```python
from build123d import *

# Parameters (mm, degrees)
F1_DEPTH = 1.85
F2_W     = 0.5
F2_H     = 21
F3_DEPTH = 3
F4_R     = 1.75
F5_DEPTH = 1.851
F6_W     = 0.25
F6_H     = 3.7
F7_DEPTH = 0.25
F8_R     = 0.24999
F9_R     = 0.4999
F10_R    = 0.24999


# Not quite as in the source:
# - a fillet or chamfer is up to 0.001 mm smaller than in the source, because OpenCascade refuses the exact size


with BuildPart() as f1:
    # F0 (on Right) → F1 (new body)
    with BuildSketch(Plane.YZ):
        Polygon((0, 9.2), (0, 0), (23.5, 0), (23.5, 13.7), (2.5, 13.7), (2.5, 9.2), align=None)
    extrude(amount=F1_DEPTH)

    # F2 (on face) → F3 (join)
    with BuildSketch(Plane.XY.offset(13.7)):
        with Locations((0.25, 13)):
            Rectangle(F2_W, F2_H)
    extrude(amount=F3_DEPTH)

    # F4 (on face) → F5 (cut, through all)
    with BuildSketch(Plane.YZ.offset(1.85)):
        with Locations((6, 3.1)):
            Circle(F4_R)
        with Locations((15, 3.1)):
            Circle(F4_R)
    extrude(amount=-F5_DEPTH, mode=Mode.SUBTRACT)

    # F6 (on face) → F7 (join)
    with BuildSketch(Plane(origin=(0, 0, 0), x_dir=(0, -1, 0), z_dir=(-1, 0, 0))):
        with Locations((-15.375, 14.85)):
            Rectangle(F6_W, F6_H)
        with Locations((-10.625, 14.85)):
            Rectangle(F6_W, F6_H)
    extrude(amount=F7_DEPTH)

    # F8 (radius 0.25 in the source; OpenCascade refuses exactly that, so slightly less here)
    f8_edges = [f1.edges().sort_by_distance(p)[0] for p in [
        (0, 6.5, 16.7),
        (0, 13, 16.7),
        (0, 19.5, 16.7),
        (0.5, 13, 16.7),
    ]]
    fillet(f8_edges, radius=F8_R)

    # F9 (radius 0.5 in the source; OpenCascade refuses exactly that, so slightly less here)
    f9_edges = [f1.edges().sort_by_distance(p)[0] for p in [
        (-0.25, 15.375, 16.7),
        (-0.25, 10.625, 16.7),
    ]]
    fillet(f9_edges, radius=F9_R)

    # F10 (radius 0.25 in the source; OpenCascade refuses exactly that, so slightly less here)
    f10_edges = [f1.edges().sort_by_distance(p)[0] for p in [
        (-0.25, 10.625, 13),
        (-0.25, 15.375, 13),
    ]]
    fillet(f10_edges, radius=F10_R)


solid = f1.part
```
For this review, take the finished solid that the model builds, in its own axes (mm). A direction names the side the tool comes from. Coordinates: 2 decimals unless noted, no trailing zeros. Write each loop counter-clockwise with the first axis right and the second up, starting at its lowest first coordinate (ties: lowest second). Pieces come first, ordered by that corner, then holes.
(1) For pin 1 Ø2 at (y, z) = (8, 15) entering from +X; pin 2 Ø3 at (y, z) = (16.5, 2) entering from -X, all flat-tipped, find the tip position at first contact; note any pin that passes through.
(2) Add section A-A on x = 0.8. Give the boundary of the cut face in (y, z), then the cut area to 3 significant figures.
(3) Wall thickness on probe 1 along Z at (x, y) = (0.6, 6); probe 2 along X at (y, z) = (16.25, 13); probe 3 along Z at (x, y) = (0.25, 2.25): over which ranges is each line inside the solid? List them lowest first.
(4) The part is to be moulded in two halves that separate along Y. For faces 4 (the face through (0.94, 4.25, 3.18)), 5 (the face through (1, 12, 0)), 6 (the face through (1, 23.5, 6)), 7 (the face through (0.938, 16.669, 3.626)), say which applies: +Y half, -Y half, draft (parallel to the pull), parting line (faces both ways), or undercut.
(5) Add section C-C on z = 3.1. Give the boundary of the cut face in (x, y), then the cut area to 3 significant figures.
(6) Tool access review of faces 1 (the face through (1, 0, 5)), 2 (the face through (1, 2.5, 12)), 3 (the face through (1, 13, 13.7)): name each direction out of +Z, -Z, +X, -X, +Y, -Y from which nothing blocks a thin tool from reaching the whole face with its end or side.
Answer sheet:
1. pin 1: stops at x = 0.5
1. pin 2: stops at x = 0
2. outline: (0, 0) - (23.5, 0) - (23.5, 13.7) - (2.5, 13.7) - (2.5, 9.2) - (0, 9.2) - close; hole circle Ø3.5 at (6, 3.1); hole circle Ø3.5 at (15, 3.1)
2. area: 291 mm2
3. probe 1: z = 0 to 1.35, 4.85 to 13.7
3. probe 2: x = 0 to 1.85
3. probe 3: z = 0 to 9.2
4. face 4: undercut
4. face 5: draft
4. face 6: +Y half
4. face 7: undercut
5. outline: (0, 0) - (1.85, 0) - (1.85, 4.25) - (0, 4.25) - close; (0, 7.75) - (1.85, 7.75) - (1.85, 13.25) - (0, 13.25) - close; (0, 16.75) - (1.85, 16.75) - (1.85, 23.5) - (0, 23.5) - close
5. area: 30.5 mm2
6. face 1: +Z, -Z, +X, -X, -Y
6. face 2: +Z, +X, -X, -Y
6. face 3: +Z, +X, +Y, -Y
